from build123d import *

# Parameters (mm, degrees)
SKETCH1_W           = 117
SKETCH1_H           = 200
BOSS_EXTRUDE1_DEPTH = 2
CUT_EXTRUDE1_DEPTH  = 2
SKETCH3_R           = 2.5
SKETCH3_R_2         = 1.5
SKETCH3_R_3         = 12.5
CUT_EXTRUDE2_DEPTH  = 30
FILLET1_R           = 20
CUT_EXTRUDE3_DEPTH  = 10
FILLET2_R           = 10
CUT_EXTRUDE4_DEPTH  = 10
FILLET3_R           = 10
CUT_EXTRUDE5_DEPTH  = 10
FILLET4_R           = 10


with BuildPart() as part:
    # Sketch1 → Boss-Extrude1 (new body)
    with BuildSketch(Plane.XY):
        with Locations((58.5, 100)):
            Rectangle(SKETCH1_W, SKETCH1_H)
    extrude(amount=BOSS_EXTRUDE1_DEPTH)

    # Sketch2 → Cut-Extrude1 (cut)
    with BuildSketch(Plane.XY.offset(2)):
        Polygon((0, 120), (40, 200), (0, 200), align=None)
        Polygon((77, 200), (117, 120), (117, 200), align=None)
    extrude(amount=-CUT_EXTRUDE1_DEPTH, mode=Mode.SUBTRACT)

    # Sketch3 → Cut-Extrude2 (cut)
    with BuildSketch(Plane.XY.offset(2)):
        with Locations((58.5, 170)):
            Circle(SKETCH3_R)
        with Locations((58.5, 150)):
            Circle(SKETCH3_R)
        with Locations((28.5, 15)):
            Circle(SKETCH3_R)
        with Locations((88.5, 15)):
            Circle(SKETCH3_R)
        with Locations((28.5, 75)):
            Circle(SKETCH3_R)
        with Locations((88.5, 75)):
            Circle(SKETCH3_R)
        with Locations((43, 112.5)):
            Circle(SKETCH3_R_2)
        with Locations((43, 81.5)):
            Circle(SKETCH3_R_2)
        with Locations((74, 81.5)):
            Circle(SKETCH3_R_2)
        with Locations((74, 112.5)):
            Circle(SKETCH3_R_2)
        with Locations((58.5, 97)):
            Circle(SKETCH3_R_3)
    extrude(amount=-CUT_EXTRUDE2_DEPTH, mode=Mode.SUBTRACT)

    # Fillet1
    fillet1_edges = [part.edges().sort_by_distance(p)[0] for p in [
        (0, 120, 1),
        (40, 200, 1),
        (117, 120, 1),
        (77, 200, 1),
        (117, 0, 1),
        (0, 0, 1),
    ]]
    fillet(fillet1_edges, radius=FILLET1_R)

    # Sketch4 → Cut-Extrude3 (cut)
    with BuildSketch(Plane(origin=(0, 0, 0), x_dir=(-1, 0, 0), z_dir=(0, 0, -1))):
        with BuildLine():
            Line((-97, 0), (-98.708203932, 156.583592135))
            Line((-98.708203932, 156.583592135), (-114.88854382, 124.22291236))
            ThreePointArc((-114.88854382, 124.22291236), (-116.464979789, 119.873698861), (-117, 115.27864045))
            Line((-117, 115.27864045), (-117, 20))
            ThreePointArc((-117, 20), (-111.142135624, 5.857864376), (-97, 0))
        make_face()
        with BuildLine():
            Line((-20, 0), (-20, 160))
            Line((-20, 160), (-18.291796068, 156.583592135))
            Line((-18.291796068, 156.583592135), (-2.11145618, 124.22291236))
            ThreePointArc((-2.11145618, 124.22291236), (-0.535020211, 119.873698861), (0, 115.27864045))
            Line((0, 115.27864045), (0, 20))
            ThreePointArc((0, 20), (-5.857864376, 5.857864376), (-20, 0))
        make_face()
    extrude(amount=-CUT_EXTRUDE3_DEPTH, mode=Mode.SUBTRACT)

    # Fillet2
    fillet2_edges = [part.edges().sort_by_distance(p)[0] for p in [
        (97, 0, 1),
        (20, 0, 1),
        (98.708203932, 156.583592135, 1),
        (20, 160, 1),
    ]]
    fillet(fillet2_edges, radius=FILLET2_R)

    # Sketch5 → Cut-Extrude4 (cut)
    with BuildSketch(Plane(origin=(0, 0, 0), x_dir=(-1, 0, 0), z_dir=(0, 0, -1))):
        with BuildLine():
            Line((-97.880566934, 80.717724073), (-77.880566934, 80.717724073))
            ThreePointArc((-77.880566934, 80.717724073), (-58.940283467, 61.777440606), (-40, 80.717724073))
            Line((-40, 80.717724073), (-20, 80.717724073))
            Line((-20, 80.717724073), (-20, 83.819660113))
            Line((-20, 83.819660113), (-20, 157.639320225))
            ThreePointArc((-20, 157.639320225), (-20.267510105, 159.93684943), (-21.05572809, 162.11145618))
            Line((-21.05572809, 162.11145618), (-34.472135955, 188.94427191))
            ThreePointArc((-34.472135955, 188.94427191), (-41.846057533, 197.013016167), (-52.360679775, 200))
            Line((-52.360679775, 200), (-64.639320225, 200))
            ThreePointArc((-64.639320225, 200), (-75.153942467, 197.013016167), (-82.527864045, 188.94427191))
            Line((-82.527864045, 188.94427191), (-97.626690246, 158.746619509))
            ThreePointArc((-97.626690246, 158.746619509), (-98.427295018, 156.518894044), (-98.681823334, 154.165397904))
            Line((-98.681823334, 154.165397904), (-97.894862718, 82.028156127))
            Line((-97.894862718, 82.028156127), (-97.880566934, 80.717724073))
        make_face()
    extrude(amount=-CUT_EXTRUDE4_DEPTH, mode=Mode.SUBTRACT)

    # Fillet3
    fillet3_edges = [part.edges().sort_by_distance(p)[0] for p in [
        (40, 80.717724073, 1),
        (77.880566934, 80.717724073, 1),
        (20, 80.717724073, 1),
        (97.880566934, 80.717724073, 1),
    ]]
    fillet(fillet3_edges, radius=FILLET3_R)

    # Sketch6 → Cut-Extrude5 (cut)
    with BuildSketch(Plane(origin=(0, 0, 0), x_dir=(-1, 0, 0), z_dir=(0, 0, -1))):
        Polygon((-58.940283467, 51.794857369), (-73.940283467, 43.134603332), (-73.940283467, 25.814095256), (-58.940283467, 17.153841218), (-43.940283467, 25.814095256), (-43.940283467, 43.134603332), align=None)
    extrude(amount=-CUT_EXTRUDE5_DEPTH, mode=Mode.SUBTRACT)

    # Fillet4
    fillet4_edges = [part.edges().sort_by_distance(p)[0] for p in [
        (58.940283467, 51.794857369, 1),
        (43.940283467, 43.134603332, 1),
        (43.940283467, 25.814095256, 1),
        (58.940283467, 17.153841218, 1),
        (73.940283467, 25.814095256, 1),
        (73.940283467, 43.134603332, 1),
    ]]
    fillet(fillet4_edges, radius=FILLET4_R)


solid = part.part
Check sheet for the modelled part. Datum: model origin and axes. Units: mm. A direction names the side the tool comes from. Give positions to 0.01 mm unless a question says otherwise; leave off trailing zeros. Loops run counter-clockwise (first coordinate to the right, second up) from the corner with the lowest first, then second, coordinate; pieces in that order, holes last. Notation, with made-up numbers: M 72,27.25 L 125,27.25 A18 ccw 125,40.25 Z; hole C -24,70.25 d7. An arc over 180 degrees is marked long. Return JSON: item names as keys, results as strings. Group by question number.
1. Cross-section at D-D on y = 15. Record the boundary of the cut face in (x, z), plus the area to 3 significant figures.
2. Cross-section at A-A on z = 0.85. Record the boundary of the cut face in (x, y).
3. Cross-section at C-C on x = 66. Record the boundary of the cut face in (y, z).
4. Mould release check, pull along X, two halves, no side actions. Record for faces 4 (the cylindrical face through (94.8, 77.83, 1.01)), 5 (the flat face through (50, 50, 0)), 6 (the flat face through (51.405, 47.445, 0.986)): released by +X, released by -X, zero draft, split by the parting line, or undercut.
5. Tool access check on faces 1 (the flat face through (73.94, 35, 1)), 2 (the cylindrical face through (37.43, 78.97, 1.01)), 3 (the cylindrical face through (94.22, 2.97, 1.01)). Record the directions out of +Z, -Z, +X, -X, +Y, -Y that give a thin tool (end or side, any length) a straight path to the whole face; none if there is none.
6. Thickness scan on L1, parallel to Y at x = 28.5, z = 0.85; L2, parallel to Y at x = 88.5, z = 1.25; L3, parallel to X at y = 13, z = 0.9. Record the ranges inside material, lowest first.
7. Cross-section at B-B on y = 65. Record the boundary of the cut face in (x, z), plus the area to 3 significant figures.
8. Go/stop test with flat-tipped pins: pin 1 (1 mm diameter, centred on y = 63.5, z = 0, fed in from +X); pin 2 (12 mm diameter, centred on x = 58, y = 38.5, fed in from +Z); pin 3 (0.6 mm diameter, centred on y = 34, z = 0.5, fed in from +X). Record where each tip stops, or that it passes through.
Return value:
{
 "1": {"outline": "M 20,0 L 26,0 L 26,2 L 20,2 Z; M 31,0 L 86,0 L 86,2 L 31,2 Z; M 91,0 L 97.16,0 L 97.16,2 L 91,2 Z", "area": "134 mm^2"},
 "2": {"outline": "M 20,10 A10 ccw 30,0 L 87.11,0 A10 ccw 97.11,9.89 L 97.77,70.61 A10 ccw 87.77,80.72 L 86.1,80.72 A10 ccw 76.71,74.17 A18.94 cw 41.17,74.17 A10 ccw 31.78,80.72 L 30,80.72 A10 ccw 20,70.72 Z; hole C 28.5,15 d5; hole C 28.5,75 d5; hole M 43.94,31.59 A10 ccw 48.94,22.93 L 53.94,20.04 A10 ccw 63.94,20.04 L 68.94,22.93 A10 ccw 73.94,31.59 L 73.94,37.36 A10 ccw 68.94,46.02 L 63.94,48.91 A10 ccw 53.94,48.91 L 48.94,46.02 A10 ccw 43.94,37.36 Z; hole C 88.5,15 d5; hole C 88.5,75 d5"},
 "3": {"outline": "M 0,0 L 21.23,0 L 21.23,2 L 0,2 Z; M 47.72,0 L 63.14,0 L 63.14,2 L 47.72,2 Z"},
 "4": {"face 4": "released by +X", "face 5": "zero draft", "face 6": "undercut"},
 "5": {"face 1": "+Z, -Z", "face 2": "+Z, -Z, +Y", "face 3": "+Z, -Z, +X, -Y"},
 "6": {"L1": "0.11 to 12.5, 17.5 to 72.5, 77.5 to 80.6", "L2": "0.1 to 12.5, 17.5 to 72.5, 77.5 to 80.69", "L3": "20 to 27, 30 to 87, 90 to 97.14"},
 "7": {"outline": "M 20,0 L 48.37,0 L 48.37,2 L 20,2 Z; M 69.51,0 L 97.71,0 L 97.71,2 L 69.51,2 Z", "area": "113 mm^2"},
 "8": {"pin 1": "x = 97.7", "pin 2": "through", "pin 3": "x = 97.37"}
}
